Autodesk Inventor part; units mm, degrees
ref_plane "YZ Plane" through (0, 0, 0) normal (1, 0, 0) x (0, 1, 0)
ref_plane "XZ Plane" through (0, 0, 0) normal (0, 1, 0) x (-1, 0, 0)
ref_plane "XY Plane" through (0, 0, 0) normal (0, 0, 1) x (1, 0, 0)
sketch "スケッチ1" plane through (0, 0, 0) normal (0, 0, 1) x (1, 0, 0)
  circle A0 centre (0, 0) radius 1.5
  dimension "d0" = 3
extrude "押し出し1" add sketch "スケッチ1" along normal blind 6
sketch "スケッチ2" plane through (0, 0, 6) normal (0, 0, 1) x (1, 0, 0)
  circle A0 centre (0, 0) radius 1.5
  circle A1 centre (0, 0) radius 3
  dimension "d3" = 6
extrude "押し出し2" add sketch "スケッチ2" along normal blind 3 contours A0 | A1
thread "ねじ1"
sketch "スケッチ4" plane through (0, 0, 0) normal (0, 0, -1) x (-1, 0, 0)
  circle A0 centre (0, 0) radius 1.5
extrude "押し出し4" cut sketch "スケッチ4" against normal blind 1.25
sketch "スケッチ5" plane through (0, 0, 1.25) normal (0, 0, -1) x (-1, 0, 0)
  circle A0 centre (0, 0) radius 1.5
extrude "押し出し5" cut sketch "スケッチ5" against normal blind 0.75
properties part number "SB　4mm ボルト" material "Steel, Mild"
The listing builds one solid part. Answer for the finished solid, in the listing's coordinates (mm). A direction names the side the tool comes from. Round coordinates to 2 decimals unless told otherwise and drop trailing zeros. Loops run counter-clockwise (first coordinate to the right, second up) from the corner with the lowest first, then second, coordinate; pieces in that order, holes last.
1) A cutting plane is placed at D-D on z = 5.75. Determine the outline of the cut face in (x, y).
Outcome:
outline: circle Ø3 at (0, 0)
2) For a pull along Y with two mould halves and no side action, classify faces 3 (the face through (-3, 0, 7)), 4 (the face through (0, 0, 2)) as released by +Y, released by -Y, zero draft, split by the parting line, or undercut.
Outcome:
face 3: split by the parting line
face 4: zero draft
3) For faces 1 (the face through (0, 0, 9)), 2 (the face through (-1.5, -0.07, 3.97)), determine the directions among +Z, -Z, +X, -X, +Y, -Y from which every point of the face is accessible in a straight line to the end or side of a thin tool.
Outcome:
face 1: +Z, +X, -X, +Y, -Y
face 2: -Z
4) A cutting plane is placed at C-C on z = 7.5. Determine the outline of the cut face in (x, y), plus the area to 3 significant figures.
Outcome:
outline: circle Ø6 at (0, 0)
area: 28.3 mm2
5) Consider line 1 (Z direction, x = 0.3, y = -2.55); line 2 (Y direction, x = 0.15, z = 8.5); line 3 (Y direction, x = 1.3, z = 7.75). Determine where each line is inside the solid, lowest interval first.
Outcome:
line 1: z = 6 to 9
line 2: y = -3 to 3
line 3: y = -2.7 to 2.7
6) Given P1, Ø1.5, axis at x = 2.5, y = -1.5, coming from the -Z side; P2, Ø1, axis at y = 2.5, z = 8, coming from the +X side, each flat-ended and moving along its own axis, determine where each tip first touches the part or whether it passes through.
Outcome:
P1: stops at z = 6
P2: stops at x = 2.24
7) A cutting plane is placed at A-A on x = 0. Determine the outline of the cut face in (y, z).
Outcome:
outline: (-3, 6) - (-1.5, 6) - (-1.5, 2) - (1.5, 2) - (1.5, 6) - (3, 6) - (3, 9) - (-3, 9) - close
